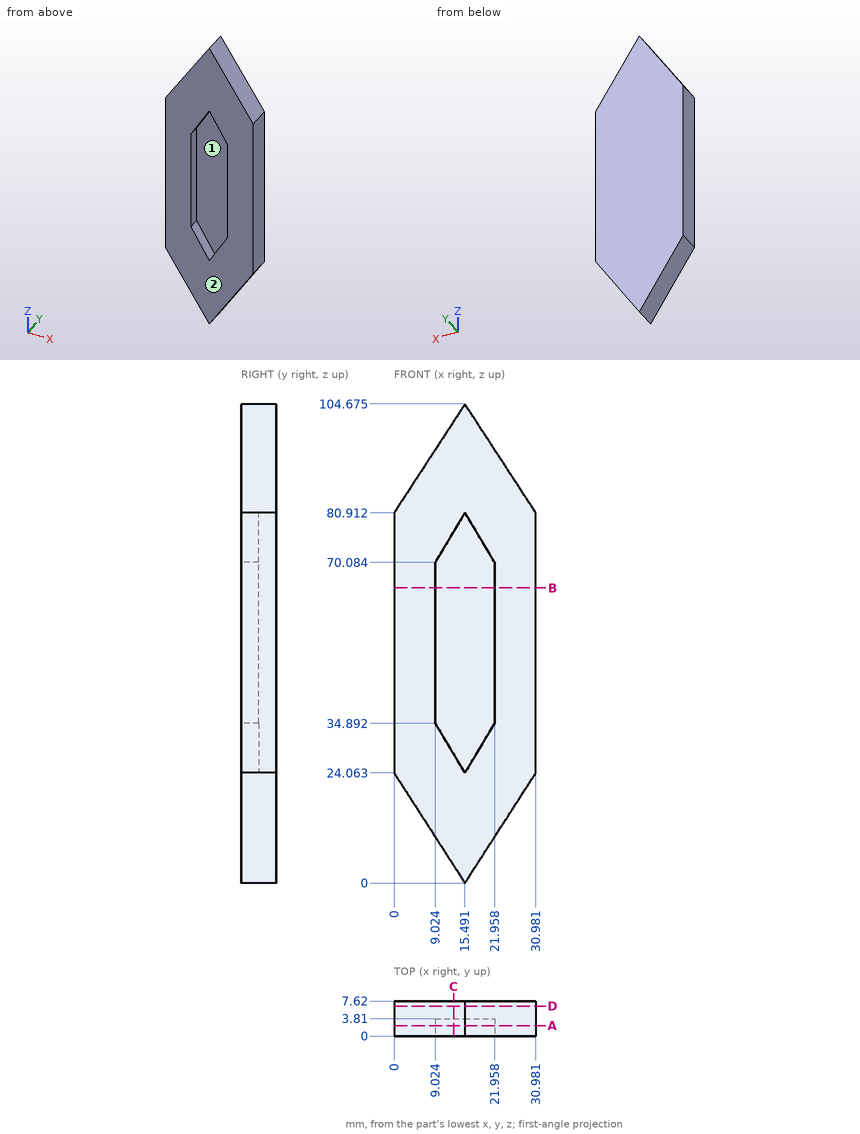
Input: dimensioned drawing with shaded views. Units: mm. Origin: part minimum x, y, z. Give positions to 0.01 mm unless a question says otherwise; leave off trailing zeros. Write each loop counter-clockwise with the first axis right and the second up, starting at its lowest first coordinate (ties: lowest second). Pieces come first, ordered by that corner, then holes. Notation, with made-up numbers: M 43,65.5 L 79,65.5 A9 ccw 79,75.5 Z; hole C 61,-35 d10. An arc over 180 degrees is marked long. Return JSON: item names as keys, results as strings. Group by question number.
1) Pull-direction query (X, two-part tool) for the marked faces 1 and 2; classes: pulls with the +X half, pulls with the -X half, needs draft (parallel to the pull), parting line crosses it, or undercut.
2) Cut plane C-C, the plane x = 13. Output: boundary loops of the cut face in (y, z).
3) Cut plane D-D, the plane y = 6.5. Output: boundary loops of the cut face in (x, z) (1 decimal).
4) Material intervals for line 1 along Z through (x, y) = (15.5, 0.5) (1 decimal); line 2 along X through (y, z) = (1.5, 39.5); line 3 along Y through (x, z) = (14.5, 56), sorted ascending. Write a range as [from, to].
5) Cut plane B-B, the plane z = 64.5. Output: boundary loops of the cut face in (x, y), plus the area to 3 significant figures.
6) Pin query (flat end, axial travel): P1, Ø1, axis at y = 6.5, z = 83, coming from the +X side; P2, Ø1.5, axis at y = 3.5, z = 21.5, coming from the -X side; P3, Ø4, axis at x = 11.5, y = 1, coming from the -Z side. Return the tip coordinate at first contact, or that it passes through.
7) Cut plane A-A, the plane y = 2.25. Output: boundary loops of the cut face in (x, z) (1 decimal), plus the area to 3 significant figures.
Recorded:
{
 "1": {"face 1": "undercut", "face 2": "needs draft"},
 "2": {"outline": "M 0,3.87 L 7.62,3.87 L 7.62,100.85 L 0,100.85 L 0,76.74 L 3.81,76.74 L 3.81,28.23 L 0,28.23 Z"},
 "3": {"outline": "M 0,24.1 L 15.5,0 L 31,24.1 L 31,80.9 L 15.5,104.7 L 0,80.9 Z"},
 "4": {"line 1": "z = [0, 24.1], [80.9, 104.7]", "line 2": "x = [0, 9.02], [21.96, 30.98]", "line 3": "y = [3.81, 7.62]"},
 "5": {"outline": "M 0,0 L 9.02,0 L 9.02,3.81 L 21.96,3.81 L 21.96,0 L 30.98,0 L 30.98,7.62 L 0,7.62 Z", "area": "187 mm²"},
 "6": {"P1": "stops at x = 29.95", "P2": "stops at x = 1.17", "P3": "stops at z = 3.09"},
 "7": {"outline": "M 0,24.1 L 15.5,0 L 31,24.1 L 31,80.9 L 15.5,104.7 L 0,80.9 Z; hole M 9,34.9 L 15.5,24.1 L 22,34.9 L 22,70.1 L 15.5,80.9 L 9,70.1 Z", "area": "1,910 mm²"}
}
